CAD build for the part. Positions are in the model's coordinates, mm. A direction names the side the tool comes from. Give positions to 0.01 mm unless a question says otherwise; leave off trailing zeros. Order: outer loops, then holes, each group sorted by start corner. A loop starts at its lowest first (then second) coordinate and runs counter-clockwise, first axis right, second up.
```python
from build123d import *

# Parameters (mm, degrees)
SKETCH1_R                = 15
BOSS_EXTRUDE1_DEPTH      = 15
SKETCH4_W                = 5
SKETCH4_H                = 33
BOSS_EXTRUDE3_DEPTH      = 30
FILLET2_R                = 2
CIRPATTERN7_COUNT        = 4
FILLET2_OF_CIRPATTERN7_R = 2
SKETCH7_R                = 1.45
CUT_EXTRUDE2_DEPTH       = 27
CIRPATTERN9_COUNT        = 4
CUT_EXTRUDE3_REACH       = 57.48
SKETCH8_W                = 12.55
SKETCH8_H                = 12.35
SKETCH9_R                = 1.45
CUT_EXTRUDE4_DEPTH       = 10
FILLET1_R                = 1


with BuildPart() as part:
    # Sketch1 → Boss-Extrude1 (new, symmetric)
    with BuildSketch(Plane.XY):
        Circle(SKETCH1_R)
    extrude(amount=BOSS_EXTRUDE1_DEPTH, both=True)

    # Sketch4 → Boss-Extrude3 (add)
    with BuildSketch(Plane.XY.offset(15)):
        with Locations((-7.5, 16.5)):
            Rectangle(SKETCH4_W, SKETCH4_H)
        with Locations((7.5, 16.5)):
            Rectangle(SKETCH4_W, SKETCH4_H)
    boss_extrude3 = extrude(amount=-BOSS_EXTRUDE3_DEPTH)

    # Fillet2
    fillet2_edges = [part.edges().sort_by_distance(p)[0] for p in [
        (-10, 11.180339887, 0),
        (-5, 14.142135624, 0),
        (10, 11.180339887, 0),
        (5, 14.142135624, 0),
    ]]
    fillet(fillet2_edges, radius=FILLET2_R)

    # CirPattern7: Boss-Extrude3 ×4 about axis
    cirpattern7_axis = Axis((0, 0, 0), (0, 0, 1))
    for i in range(1, CIRPATTERN7_COUNT):
        add(boss_extrude3.rotate(cirpattern7_axis, i * 360 / CIRPATTERN7_COUNT))

    # Fillet2 of CirPattern7
    fillet2_of_cirpattern7_edges = [part.edges().sort_by_distance(p)[0] for p in [
        (-11.180339887, -10, 0),
        (-14.142135624, -5, 0),
        (-11.180339887, 10, 0),
        (-14.142135624, 5, 0),
        (10, -11.180339887, 0),
        (5, -14.142135624, 0),
        (-10, -11.180339887, 0),
        (-5, -14.142135624, 0),
        (11.180339887, 10, 0),
        (14.142135624, 5, 0),
        (11.180339887, -10, 0),
        (14.142135624, -5, 0),
    ]]
    fillet(fillet2_of_cirpattern7_edges, radius=FILLET2_OF_CIRPATTERN7_R)

    # Sketch7 → Cut-Extrude2 (cut)
    with BuildSketch(Plane.ZY.offset(10)):
        with Locations((-7.5, 24)):
            Circle(SKETCH7_R)
        with Locations((7.5, 24)):
            Circle(SKETCH7_R)
        with Locations((22.5, 24)):
            Circle(SKETCH7_R)
        with Locations((37.5, 24)):
            Circle(SKETCH7_R)
        with Locations((52.5, 24)):
            Circle(SKETCH7_R)
    cut_extrude2 = extrude(amount=-CUT_EXTRUDE2_DEPTH, mode=Mode.SUBTRACT)

    # CirPattern9: Cut-Extrude2 ×4 about axis
    cirpattern9_axis = Axis((0, 0, 0), (0, 0, 1))
    for i in range(1, CIRPATTERN9_COUNT):
        add(cut_extrude2.rotate(cirpattern9_axis, i * 360 / CIRPATTERN9_COUNT), mode=Mode.SUBTRACT)

    # Sketch8 → Cut-Extrude3 (cut, up to next)
    with BuildSketch(Plane.XY.offset(15), mode=Mode.PRIVATE) as cut_extrude3_sk1:
        Rectangle(SKETCH8_W, SKETCH8_H)
    cut_extrude3_tool1 = extrude(cut_extrude3_sk1.sketch, amount=-CUT_EXTRUDE3_REACH, mode=Mode.PRIVATE) & part.part
    add(cut_extrude3_tool1.solids().sort_by_distance((0, 0, 15))[0], mode=Mode.SUBTRACT)

    # Sketch9 → Cut-Extrude4 (cut)
    with BuildSketch(Plane.XY.offset(15)):
        with Locations((10.6375, 0)):
            Circle(SKETCH9_R)
        with Locations((0, -10.5375)):
            Circle(SKETCH9_R)
        with Locations((-10.5375, 0.1)):
            Circle(SKETCH9_R)
        with Locations((0.1, 10.6375)):
            Circle(SKETCH9_R)
    cut_extrude4 = extrude(amount=-CUT_EXTRUDE4_DEPTH, mode=Mode.SUBTRACT)

    # Fillet1
    fillet1_edges = [part.edges().sort_by_distance(p)[0] for p in [
        (6.275, 6.175, 0),
        (6.275, -6.175, 0),
        (-6.275, -6.175, 0),
        (-6.275, 6.175, 0),
    ]]
    fillet(fillet1_edges, radius=FILLET1_R)

    # Mirror1: Cut-Extrude4 across plane
    add(cut_extrude4.mirror(Plane.XY), mode=Mode.SUBTRACT)


solid = part.part
```
Item 1: Wall check: L1, parallel to X at y = 6.5, z = -7.5; L2, parallel to Z at x = -24, y = 8. Give the ranges that are in metal, low to high.
Item 2: Tool access for faces 1 (the face through (-5, -25, 0)), 2 (the face through (0, 6.175, 0)), 3 (the face through (11.977, -0.555, -10.07)), 4 (the face through (25, 5, 0)), 5 (the face through (0, -11, 5)): list every direction of +Z, -Z, +X, -X, +Y, -Y with a clear straight run to the whole face (end or side of a thin tool).
Item 3: Drop flat-ended pins along their axis: pin 1 Ø8 at (y, z) = (-28, 3.5) entering from -X; pin 2 Ø2.5 at (x, z) = (-24, 7.5) entering from +Y; pin 3 Ø10.5 at (x, z) = (27, -7) entering from -Y; pin 4 Ø1.7 at (x, y) = (0.1, 10.64) entering from +Z. Give the stop position or say it passes through.
Item 4: Slice it at A-A (x = -24). Give the cut face in (y, z).
Item 5: Slice it at D-D (z = 7.5). State how many separate pieces and enclosed holes the cut face has, and give its area (3 significant figures).
Item 6: Two-plate mould, pull along X, no slides. Class faces 6 (the face through (-7, -33, 0)), 7 (the face through (10, 22, 0)), 8 (the face through (4, 15, 0)): released by +X, released by -X, zero draft, split by the parting line, or undercut.
Item 7: Slice it at B-B (x = 27). Give the cut face in (y, z).
A:
1. L1: x = -33 to -25.45, -22.55 to 22.55, 25.45 to 33
1. L2: z = -15 to -8.95, -6.05 to 6.05, 8.95 to 15
2. face 1: +Z, -Z, -Y
2. face 2: +Z, -Z
2. face 3: -Z
2. face 4: +Z, -Z, +X
2. face 5: +Z
3. pin 1: stops at x = -10
3. pin 2: passes through
3. pin 3: stops at y = -10
3. pin 4: stops at z = 5
4. outline: (-10, -15) - (-5, -15) - (-5, -8.95) - (-10, -8.95) - close; (-10, -6.05) - (-5, -6.05) - (-5, 6.05) - (-10, 6.05) - close; (-10, 8.95) - (-5, 8.95) - (-5, 15) - (-10, 15) - close; (5, -15) - (10, -15) - (10, -8.95) - (5, -8.95) - close; (5, -6.05) - (10, -6.05) - (10, 6.05) - (5, 6.05) - close; (5, 8.95) - (10, 8.95) - (10, 15) - (5, 15) - close
5. separate pieces: 9
5. enclosed holes: 5
5. area: 1,230 mm2
6. face 6: zero draft
6. face 7: released by +X
6. face 8: undercut
7. outline: (-10, -15) - (-5, -15) - (-5, 15) - (-10, 15) - close; (5, -15) - (10, -15) - (10, 15) - (5, 15) - close
